The model under review builds one solid part; all positions refer to its coordinate system, in mm. Coordinates: 2 decimals unless noted, no trailing zeros. Loops run counter-clockwise (first coordinate to the right, second up) from the corner with the lowest first, then second, coordinate; pieces in that order, holes last. Notation, with made-up numbers: (68, 71) - (127, 71) arc R33 ccw to (127, 102) - close; hole circle Ø7 at (1, 41). An arc over 180 degrees is marked (long way). Use a Markdown table: item, result. Add a question column.
1) Add section C-C, the plane z = 38. Give the boundary of the cut face in (x, y).
2) Add section D-D, the plane z = -36.5. Give the boundary of the cut face in (x, y).
3) Add section B-B, the plane z = 15.24. Give the boundary of the cut face in (x, y).
4) To check wall thickness, follow L1, parallel to Y at x = -0.1, z = -15.24; L2, parallel to Z at x = -0.35, y = 6.25; L3, parallel to Y at x = 0.45, z = 13.5. State the ranges of each line that lie inside material, in increasing order. Write a range as [from, to].
5) Clearance check with flat-ended pins moving along their axes: pin 1 (4 mm diameter, centred on y = 0, z = 37.15, fed in from -X); pin 2 (6.5 mm diameter, centred on y = -7.43, z = 15.24, fed in from -X); pin 3 (1 mm diameter, centred on x = -0.5, y = -2, fed in from -Z). State where each tip first meets the part, or that it passes through.
6) The part is to be moulded in two halves that separate along Z. For faces 1 (the cylindrical face through (-0.014, 9.455, -15.689)), 2 (the flat face through (0.014, -10.563, 32.899)), 3 (the flat face through (1, -3, -1)), say which applies: pulls with the +Z half, pulls with the -Z half, needs draft (parallel to the pull), parting line crosses it, or undercut.
7) Add section A-A, the plane y = 0. Give the boundary of the cut face in (x, z) (3 decimals), and give its area (3 significant figures).
```python
from build123d import *

# Parameters (mm, degrees)
SKETCH1_R               = 2.07
SKETCH1_R_2             = 2.5375
BOSS_EXTRUDE1_DEPTH     = 1
CUT_EXTRUDE1_DEPTH      = 48.733959609
CUT_EXTRUDE1_DEPTH_BACK = 48.733959609
FILLET1_R               = 0.250000008


with BuildPart() as part:
    # Sketch1 → Boss-Extrude1 (new, symmetric)
    with BuildSketch(Plane(origin=(0, 0, 0), x_dir=(0, 0, -1), z_dir=(1, 0, 0))):
        with BuildLine():
            Line((-26.035, 12.7), (26.035, 12.7))
            Line((26.035, 12.7), (39.770143518, 8.423671838))
            ThreePointArc((39.770143518, 8.423671838), (45.97, 0), (39.770143518, -8.423671838))
            Line((39.770143518, -8.423671838), (26.035, -12.7))
            Line((26.035, -12.7), (-26.035, -12.7))
            Line((-26.035, -12.7), (-39.770143518, -8.423671838))
            ThreePointArc((-39.770143518, -8.423671838), (-45.97, 0), (-39.770143518, 8.423671838))
            Line((-39.770143518, 8.423671838), (-26.035, 12.7))
        make_face()
        Circle(SKETCH1_R, mode=Mode.SUBTRACT)
        with Locations((-15.24, 7.434146341)):
            Circle(SKETCH1_R, mode=Mode.SUBTRACT)
        with Locations((-15.24, -7.434146341)):
            Circle(SKETCH1_R, mode=Mode.SUBTRACT)
        with Locations(Location((15.24, -7.434146341, 0), (0, 0, 180))):
            Circle(SKETCH1_R, mode=Mode.SUBTRACT)
        with Locations(Location((15.24, 7.434146341, 0), (0, 0, 180))):
            Circle(SKETCH1_R, mode=Mode.SUBTRACT)
        with Locations((-37.1475, 0)):
            Circle(SKETCH1_R_2, mode=Mode.SUBTRACT)
        with Locations(Location((37.1475, 0, 0), (0, 0, 180))):
            Circle(SKETCH1_R_2, mode=Mode.SUBTRACT)
    extrude(amount=BOSS_EXTRUDE1_DEPTH, both=True)

    # Sketch2 → Cut-Extrude1 (cut, two sides: drawn at the far end of the back side and taken through both)
    with BuildSketch(Plane(origin=(1, 0, 0), x_dir=(0, 0, -1), z_dir=(1, 0, 0)).offset(-CUT_EXTRUDE1_DEPTH_BACK)):
        with BuildLine():
            Line((-25.4, 12.7), (-25.4, 12.044028029))
            ThreePointArc((-25.4, 12.044028029), (-25.472087861, 11.948002447), (-25.58441825, 11.99042244))
            Line((-25.58441825, 11.99042244), (-26.035, 12.7))
            Line((-26.035, 12.7), (-25.4, 12.7))
        make_face()
        with BuildLine():
            Line((25.4, 12.7), (25.4, 12.044028029))
            ThreePointArc((25.4, 12.044028029), (25.472087861, 11.948002447), (25.58441825, 11.99042244))
            Line((25.58441825, 11.99042244), (26.035, 12.7))
            Line((26.035, 12.7), (25.4, 12.7))
        make_face()
        with BuildLine():
            Line((25.4, -12.7), (26.035, -12.7))
            Line((26.035, -12.7), (25.58441825, -11.99042244))
            ThreePointArc((25.58441825, -11.99042244), (25.472087861, -11.948002447), (25.4, -12.044028029))
            Line((25.4, -12.044028029), (25.4, -12.7))
        make_face()
        with BuildLine():
            Line((-25.4, -12.7), (-25.4, -12.044028029))
            ThreePointArc((-25.4, -12.044028029), (-25.472087861, -11.948002447), (-25.58441825, -11.99042244))
            Line((-25.58441825, -11.99042244), (-26.035, -12.7))
            Line((-26.035, -12.7), (-25.4, -12.7))
        make_face()
        with BuildLine():
            Line((-0.5, 12.7), (0.5, 12.7))
            Line((0.5, 12.7), (0.089442719, 11.878885438))
            ThreePointArc((0.089442719, 11.878885438), (0, 11.823606798), (-0.089442719, 11.878885438))
            Line((-0.089442719, 11.878885438), (-0.5, 12.7))
        make_face()
        with BuildLine():
            Line((-0.5, -12.7), (0.5, -12.7))
            Line((0.5, -12.7), (0.089442719, -11.878885438))
            ThreePointArc((0.089442719, -11.878885438), (0, -11.823606798), (-0.089442719, -11.878885438))
            Line((-0.089442719, -11.878885438), (-0.5, -12.7))
        make_face()
    extrude(amount=CUT_EXTRUDE1_DEPTH + CUT_EXTRUDE1_DEPTH_BACK, mode=Mode.SUBTRACT)

    # Fillet1
    fillet1_edges = [part.edges().sort_by_distance(p)[0] for p in [
        (0, -12.7, -0.5),
        (0, -12.7, 0.5),
        (0, 12.7, 0.5),
        (0, 12.7, -0.5),
        (0, 12.7, 25.4),
        (0, -12.7, -26.035),
        (0, -12.7, 26.035),
        (0, 12.7, 26.035),
        (0, 12.7, -26.035),
        (0, 12.7, -25.4),
        (0, -12.7, -25.4),
        (0, -12.7, 25.4),
    ]]
    fillet(fillet1_edges, radius=FILLET1_R)


solid = part.part
```
From the geometry:
| question | item | result |
|---|---|---|
| 1 | outline | (-1, -8.97) - (1, -8.97) - (1, -2.39) - (-1, -2.39) - close; (-1, 2.39) - (1, 2.39) - (1, 8.97) - (-1, 8.97) - close |
| 2 | outline | (-1, -9.44) - (1, -9.44) - (1, -2.45) - (-1, -2.45) - close; (-1, 2.45) - (1, 2.45) - (1, 9.44) - (-1, 9.44) - close |
| 3 | outline | (-1, -12.7) - (1, -12.7) - (1, -9.5) - (-1, -9.5) - close; (-1, -5.36) - (1, -5.36) - (1, 5.36) - (-1, 5.36) - close; (-1, 9.5) - (1, 9.5) - (1, 12.7) - (-1, 12.7) - close |
| 4 | L1 | y = [-12.7, -9.5], [-5.36, 5.36], [9.5, 12.7] |
| 4 | L2 | z = [-43.37, -16.94], [-13.54, 13.54], [16.94, 43.37] |
| 4 | L3 | y = [-12.7, -8.56], [-6.31, 6.31], [8.56, 12.7] |
| 5 | pin 1 | passes through |
| 5 | pin 2 | stops at x = -1 |
| 5 | pin 3 | stops at z = -45.84 |
| 6 | face 1 | undercut |
| 6 | face 2 | pulls with the +Z half |
| 6 | face 3 | needs draft |
| 7 | outline | (-1, -45.97) - (1, -45.97) - (1, -39.685) - (-1, -39.685) - close; (-1, -34.61) - (1, -34.61) - (1, -2.07) - (-1, -2.07) - close; (-1, 2.07) - (1, 2.07) - (1, 34.61) - (-1, 34.61) - close; (-1, 39.685) - (1, 39.685) - (1, 45.97) - (-1, 45.97) - close |
| 7 | area | 155 mm^2 |
